Here's how the part is built. I have some questions about the finished solid (model axes, mm). A direction names the side the tool comes from. Coordinates: 2 decimals unless noted, no trailing zeros. Write each loop counter-clockwise with the first axis right and the second up, starting at its lowest first coordinate (ties: lowest second). Pieces come first, ordered by that corner, then holes.
Item 1: If we section it at B-B (x = 13.5): Please give me the cut outline in (y, z) (3 decimals), then the cut area to 3 significant figures.
Item 2: For faces 4 (the face through (-4.92, -60.51, 1.57)), 5 (the face through (-32.19, -15.52, 1.57)), 6 (the face through (-30.13, 24.26, 1.21)), 7 (the face through (31.872, 4.337, 1.212)), 8 (the face through (15, 0.809, 2)), which set-ups out of +Z, -Z, +X, -X, +Y, -Y let a thin tool reach every point of the face, with its end or its side?
Item 3: If we section it at D-D (y = 16): Please give me the cut outline in (x, z) (3 decimals).
Item 4: If we section it at C-C (x = -13.5): Please give me the cut outline in (y, z) (3 decimals), then the cut area to 3 significant figures.
Item 5: If we section it at A-A (z = 2.05): Count the separate pieces of the cut face and the enclosed holes in it, then the cut area to 3 significant figures.
Item 6: If I drill on line 1 (X direction, y = -28.5, z = 0.9); line 2 (Y direction, x = 10.5, z = 0.45); line 3 (Y direction, x = 13.5, z = 2.15), over which ranges is the centre line in solid material (lowest first)?
Item 7: I'm going to push a flat-ended pin straight in: pin 1 Ø1 at (x, z) = (16, 1) entering from -Y. Where does the tip first touch, or does it pass through?
Item 8: We'd pull the mould along X, two halves only. Please class faces 1 (the face through (29.39, -39.714, 1.565)), 2 (the face through (3.43, 45.11, 1.61)), 3 (the face through (-18.84, -51.55, 1.89)): +X half, -X half, draft (parallel to the pull), parting line (faces both ways), or undercut.
from build123d import *

# Parameters (mm, degrees)
BOSS_EXTRUDE2_DEPTH = 3.175
CHAMFER3_SIZE       = 2.6
SKETCH3_R           = 8
SKETCH3_R_2         = 3.03324197
SKETCH3_R_3         = 6.375
SKETCH3_W           = 17
SKETCH3_H           = 14
CUT_EXTRUDE1_DEPTH  = 10


with BuildPart() as part:
    # Sketch2 → Boss-Extrude2 (new body)
    with BuildSketch(Plane.XY):
        Polygon((33.967630838, -35.823456397), (25.63439182, 59.425901431), (0, 64.888689731), (-25.63439182, 59.425901431), (-33.967630838, -35.823456397), (0, -64.691310269), align=None)
        Polygon((-30.464841537, 4.213608519), (-28.721726682, 24.137502481), (-32.407647065, 24.459978729), (-34.15076192, 4.536084767), align=None)
        Polygon((32.407647065, 24.459978729), (28.721726682, 24.137502481), (30.464841537, 4.213608519), (34.15076192, 4.536084767), align=None)
        Polygon((27.2046006, -46.164342336), (24.938042288, -43.497375254), (9.698230388, -56.449137036), (11.9647887, -59.116104119), align=None)
        Polygon((-9.698230388, -56.449137036), (-24.938042288, -43.497375254), (-27.2046006, -46.164342336), (-11.9647887, -59.116104119), align=None)
    extrude(amount=BOSS_EXTRUDE2_DEPTH)

    # Chamfer3
    chamfer3_edges = [part.edges().sort_by_distance(p)[0] for p in [
        (19.58469465, -52.640223227, 3.175),
        (33.279204493, 14.498031748, 3.175),
        (-33.279204493, 14.498031748, 3.175),
        (-19.58469465, -52.640223227, 3.175),
    ]]
    chamfer(chamfer3_edges, length=CHAMFER3_SIZE)

    # Sketch3 → Cut-Extrude1 (cut)
    with BuildSketch(Plane.XY.offset(3.175)):
        with Locations((13.5, -30.691310269)):
            Circle(SKETCH3_R)
        with Locations((-13.5, -30.691310269)):
            Circle(SKETCH3_R)
        with Locations((0, -11.191310269)):
            Circle(SKETCH3_R_2)
        with Locations((0, 39.734509442)):
            Circle(SKETCH3_R_3)
        with Locations((15.5, 7.808689731)):
            Rectangle(SKETCH3_W, SKETCH3_H)
    extrude(amount=-CUT_EXTRUDE1_DEPTH, mode=Mode.SUBTRACT)


solid = part.part
Answer list:
1. outline: (-57.811, 0) - (-38.691, 0) - (-38.691, 3.175) - (-54.399, 3.175) - (-57.811, 0.575) - close; (-22.691, 0) - (0.809, 0) - (0.809, 3.175) - (-22.691, 3.175) - close; (14.809, 0) - (62.012, 0) - (62.012, 3.175) - (14.809, 3.175) - close
1. area: 281 mm2
2. face 4: +Z, -Z, -Y
2. face 5: +Z, -Z, -X
2. face 6: +Z, -Z, +Y
2. face 7: +Z, -Z, +X
2. face 8: +Z, -Z
3. outline: (-33.148, 0) - (33.148, 0) - (33.148, 0.575) - (30.538, 3.175) - (-30.538, 3.175) - (-33.148, 0.575) - close
4. outline: (-57.811, 0) - (-38.691, 0) - (-38.691, 3.175) - (-54.399, 3.175) - (-57.811, 0.575) - close; (-22.691, 0) - (62.012, 0) - (62.012, 3.175) - (-22.691, 3.175) - close
4. area: 325 mm2
5. separate pieces: 1
5. enclosed holes: 5
5. area: 6,170 mm2
6. line 1: x = -33.33 to -21.19, -5.81 to 5.81, 21.19 to 33.33
6. line 2: y = -57.39 to -38.11, -23.28 to 0.81, 14.81 to 62.65
6. line 3: y = -55.74 to -38.69, -22.69 to 0.81, 14.81 to 62.01
7. pin 1: stops at y = -55.91
8. face 1: +X half
8. face 2: undercut
8. face 3: -X half
